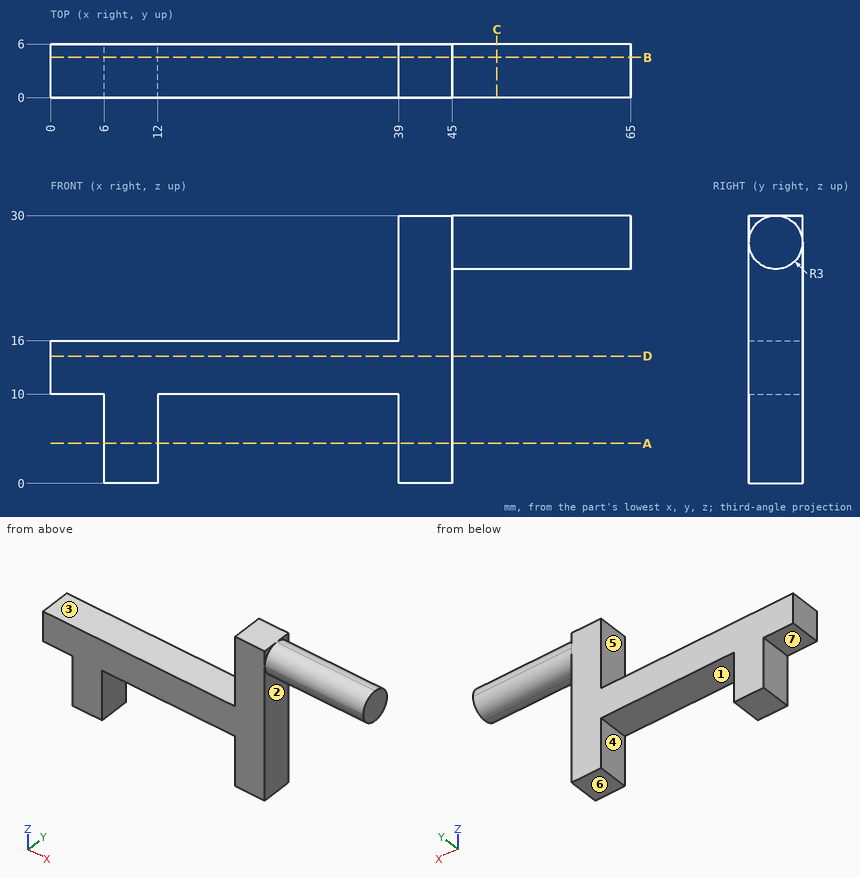
Could you check a few things on this drawing? It's one solid part, dimensions in mm from its lowest x, y, z. A direction names the side the tool comes from. Give positions to 0.01 mm unless a question says otherwise; leave off trailing zeros. Order: outer loops, then holes, each group sorted by start corner. A loop starts at its lowest first (then second) coordinate and runs counter-clockwise, first axis right, second up. Notation, with made-up numbers: M 23,78 L 71,78 A24 cw 71,104 Z; hole C -25.75,32.25 d11. An arc over 180 degrees is marked long. Use one line per item in the form item = value.
Item 1: If we section it at D-D, the plane z = 14.25: Write out the boundary of the cut face in (x, y), and give its area (3 significant figures).
Values follow:
outline = M 0,0 L 45,0 L 45,6 L 0,6 Z
area = 270 mm^2
Item 2: If we section it at C-C, the plane x = 50: Write out the boundary of the cut face in (y, z), and give its area (3 significant figures).
Values follow:
outline = C 3,27 d6
area = 28.3 mm^2
Item 3: If we section it at A-A, the plane z = 4.5: Write out the boundary of the cut face in (x, y), and give its area (3 significant figures).
Values follow:
outline = M 6,0 L 12,0 L 12,6 L 6,6 Z; M 39,0 L 45,0 L 45,6 L 39,6 Z
area = 72.0 mm^2
Item 4: If we section it at B-B, the plane y = 4.5: Write out the boundary of the cut face in (x, z), and give its area (3 significant figures).
Values follow:
outline = M 0,10 L 6,10 L 6,0 L 12,0 L 12,10 L 39,10 L 39,0 L 45,0 L 45,24.4 L 65,24.4 L 65,29.6 L 45,29.6 L 45,30 L 39,30 L 39,16 L 0,16 Z
area = 578 mm^2
Item 5: Thinking about a two-plate mould opening in X: for the marked faces 1, 2 and 3, which applies, pulls with the +X half, pulls with the -X half, needs draft (parallel to the pull), parting line crosses it, or undercut?
Values follow:
face_1 = undercut
face_2 = pulls with the +X half
face_3 = needs draft
Item 6: If I drill on line 1 along X through (y, z) = (2.75, 3.5); line 2 along Z through (x, y) = (27, 5.5); line 3 along X through (y, z) = (5.25, 10.5), over which ranges is the centre line in solid material (lowest first)? Write a range as [from, to].
Values follow:
line_1 = [6, 12], [39, 45]
line_2 = [10, 16]
line_3 = [0, 45]
Item 7: Will these pins go through, and if not, where does the flat tip stop? pin 1 Ø3 at (x, y) = (21.5, 3) entering from +Z; pin 2 Ø1.8 at (x, y) = (31, 4) entering from -Z; pin 3 Ø10 at (x, z) = (54.5, 21) entering from +Y.
Values follow:
pin_1 = 16
pin_2 = 10
pin_3 = 5.83
Item 8: For the marked faces 4, 5, 6 and 7, which set-ups out of +Z, -Z, +X, -X, +Y, -Y let a thin tool reach every point of the face, with its end or its side?
Values follow:
face_4 = -Z, +Y, -Y
face_5 = +Z, -X, +Y, -Y
face_6 = -Z, +X, -X, +Y, -Y
face_7 = -Z, -X, +Y, -Y
